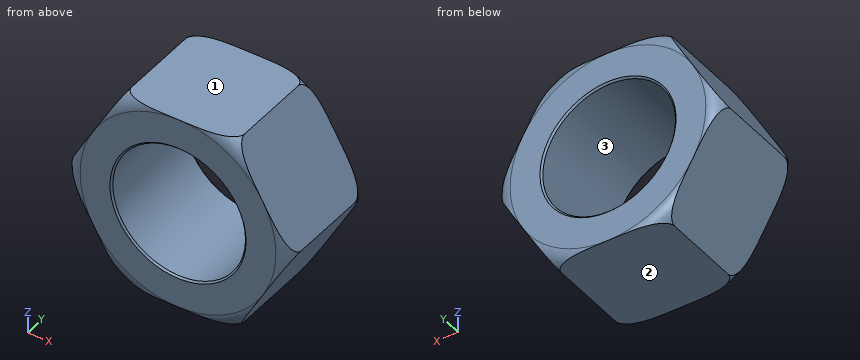
```python
from build123d import *

# Parameters (mm, degrees)
BOSS_EXTRUDE1_DEPTH = 64
SKETCH6_R           = 78
CUT_EXTRUDE1_DEPTH  = 129.000000101
CHAMFER1_SIZE       = 2


with BuildPart() as part:
    # Sketch1 → Boss-Extrude1 (new body, symmetric)
    with BuildSketch(Plane(origin=(0, 0, 0), x_dir=(1, 0, 0), z_dir=(0, 1, 0))):
        Polygon((132.790561914, 0), (66.395280957, 115), (-66.395280957, 115), (-132.790561914, 0), (-66.395280957, -115), (66.395280957, -115), align=None)
    extrude(amount=BOSS_EXTRUDE1_DEPTH, both=True)

    # Sketch3 → Cut-Revolve1 (revolve, cut)
    with BuildSketch(Plane.XY):
        with BuildLine():
            Line((-132.790561914, 64), (-132.790561914, 46.209438086))
            ThreePointArc((-132.790561914, 46.209438086), (-127.57982697, 58.789265057), (-115, 64))
            Line((-115, 64), (-132.790561914, 64))
        make_face()
    cut_revolve1 = revolve(axis=Axis((0, -11.068960952, 0), (0, -1, 0)), mode=Mode.SUBTRACT)

    # Mirror1: Cut-Revolve1 across plane
    add(cut_revolve1.mirror(Plane.ZX), mode=Mode.SUBTRACT)

    # Sketch6 → Cut-Extrude1 (cut, through all)
    with BuildSketch(Plane(origin=(0, 64, 0), x_dir=(1, 0, 0), z_dir=(0, 1, 0))):
        Circle(SKETCH6_R)
    extrude(amount=-CUT_EXTRUDE1_DEPTH, mode=Mode.SUBTRACT)

    # Chamfer1
    chamfer1_edges = [part.edges().sort_by_distance(p)[0] for p in [
        (-78, -64, 0),
        (-78, 64, 0),
    ]]
    chamfer(chamfer1_edges, length=CHAMFER1_SIZE)


solid = part.part
```
For this review, take the finished solid that the model builds, in its own axes (mm). Face numbers are marked on the shaded views. Coordinates: 2 decimals unless noted, no trailing zeros. Order: outer loops, then holes, each group sorted by start corner. A loop starts at its lowest first (then second) coordinate and runs counter-clockwise, first axis right, second up. Notation, with made-up numbers: (-34.5, 81.5) - (-16.5, 81.5) arc R11 ccw to (-16.5, 96.5) - close; hole circle Ø4 at (77.25, -37). An arc over 180 degrees is marked (long way). Answer as a JSON object with one key per item and string values. Group by question number.
1. Clearance check with flat-ended pins moving along their axes: P1, Ø2, axis at y = -29, z = -90, coming from the +X side; P2, Ø2, axis at y = 6, z = -83.5, coming from the -X side; P3, Ø10, axis at x = 90, y = -34, coming from the -Z side. State where each tip first meets the part, or that it passes through.
2. For probe 1 along X at (y, z) = (31, 0); probe 2 along X at (y, z) = (-59, 65); probe 3 along Z at (x, y) = (6, 34.5), list the stretches that pass through material, from the lowest coordinate up.
3. We need section A-A on y = 8. State the section outline as (x, z) points, then the cut area to 3 significant figures.
4. The part is to be moulded in two halves that separate along Z. For the marked faces 1, 2 and 3, say which applies: pulls with the +Z half, pulls with the -Z half, needs draft (parallel to the pull), parting line crosses it, or undercut.
Final values:
{
 "1": {"P1": "x = 81.41", "P2": "x = -85.16", "P3": "z = -82.78"},
 "2": {"probe 1": "-132.79 to -78, 78 to 132.79", "probe 2": "-95.26 to -43.12, 43.12 to 95.26", "probe 3": "-115 to -77.77, 77.77 to 115"},
 "3": {"outline": "(-132.79, 0) - (-66.4, -115) - (66.4, -115) - (132.79, 0) - (66.4, 115) - (-66.4, 115) - close; hole circle Ø156 at (0, 0)", "area": "26,700 mm²"},
 "4": {"face 1": "pulls with the +Z half", "face 2": "pulls with the -Z half", "face 3": "undercut"}
}
